```python
from build123d import *

# Parameters (mm, degrees)
F1_DEPTH = 12
F2_R     = 2.75
F3_DEPTH = 25
F4_R     = 4
F5_R     = 2
F6_R     = 1.6
F7_DEPTH = 25.001


with BuildPart() as f1:
    # F0 (on Top) → F1 (new body)
    with BuildSketch(Plane.XY):
        with BuildLine():
            ThreePointArc((1, 3.872983), (0, -4), (-1, 3.872983))
            Line((-1, 3.872983), (-1, 6.928203))
            Line((-1, 6.928203), (-1, 9.872983))
            Line((-1, 9.872983), (-5, 9.872983))
            Line((-5, 9.872983), (-5, 4.898979))
            ThreePointArc((-5, 4.898979), (-6.480741, 2.645751), (-7, 0))
            Line((-7, 0), (-7, -19))
            Line((-7, -19), (-20, -19))
            Line((-20, -19), (-20, -23))
            Line((-20, -23), (0, -23))
            Line((0, -23), (20, -23))
            Line((20, -23), (20, -19))
            Line((20, -19), (7, -19))
            Line((7, -19), (7, 0))
            ThreePointArc((7, 0), (6.480741, 2.645751), (5, 4.898979))
            Line((5, 4.898979), (5, 9.872983))
            Line((5, 9.872983), (1, 9.872983))
            Line((1, 9.872983), (1, 6.872983))
            Line((1, 6.872983), (1, 3.872983))
        make_face()
    extrude(amount=F1_DEPTH)

    # F2 (on face) → F3 (cut)
    with BuildSketch(Plane(origin=(0, -19, 0), x_dir=(-1, 0, 0), z_dir=(0, 1, 0))):
        with Locations((-13.5, 6)):
            Circle(F2_R)
        with Locations((13.5, 6)):
            Circle(F2_R)
    extrude(amount=-F3_DEPTH, mode=Mode.SUBTRACT)

    # F4
    f4_edges = [f1.edges().sort_by_distance(p)[0] for p in [
        (20, -21, 12),
        (20, -21, 0),
        (-20, -21, 0),
        (-20, -21, 12),
    ]]
    fillet(f4_edges, radius=F4_R)

    # F5
    f5_edges = [f1.edges().sort_by_distance(p)[0] for p in [
        (7, -19, 6),
        (-7, -19, 6),
    ]]
    fillet(f5_edges, radius=F5_R)

    # F6 (on face) → F7 (cut, through all)
    with BuildSketch(Plane.YZ.offset(5)):
        with Locations((7.385981, 6)):
            Circle(F6_R)
    extrude(amount=-F7_DEPTH, mode=Mode.SUBTRACT)


solid = f1.part
```
Geometry: final body of the model. Coordinates: model frame, mm. A direction names the side the tool comes from. Round coordinates to 2 decimals unless told otherwise and drop trailing zeros. Write each loop counter-clockwise with the first axis right and the second up, starting at its lowest first coordinate (ties: lowest second). Pieces come first, ordered by that corner, then holes.
Item 1: Section query B-B (z = 6). Give the number of separate pieces and of enclosed holes in the cut face, plus the area to 3 significant figures.
Item 2: Section query C-C (y = -1). Return loops of the section in (x, z), plus the area to 3 significant figures.
Item 3: Material intervals for L1, parallel to X at y = 0, z = 5.5; L2, parallel to Z at x = 13.5, y = -21.55; L3, parallel to X at y = 6, z = 1, sorted ascending.
Item 4: Section query D-D (x = 1.5). Return loops of the section in (y, z), plus the area to 3 significant figures.
Item 5: Mould query, pull axis X, two halves, no side actions, for faces 4 (the face through (1, 5.6, 5.9)), 5 (the face through (6.5, 2.6, 5.9)), 6 (the face through (0, -23, 6)), 7 (the face through (-1, 5, 6)). Classes: +X half, -X half, draft (parallel to the pull), parting line (faces both ways), or undercut.
Item 6: Section query A-A (x = 13.5). Return loops of the section in (y, z), plus the area to 3 significant figures.
Item 7: Set-up query: faces 1 (the face through (0, -10, 0)), 2 (the face through (17, -19, 6)), 3 (the face through (-5, 6.3, 4.6)). Return all of +Z, -Z, +X, -X, +Y, -Y with unobstructed straight access to the full face (end or side cutting, diameter ignored); none if empty.
Item 8: Pin query (flat end, axial travel): P1, Ø1.8, axis at y = 7.5, z = 8, coming from the -X side; P2, Ø1.5, axis at y = -4, z = 9.5, coming from the +X side; P3, Ø5.5, axis at x = -15, z = 5, coming from the +Y side. Return the tip coordinate at first contact, or that it passes through.
Completed:
1. separate pieces: 5
1. enclosed holes: 0
1. area: 408 mm2
2. outline: (-7, 0) - (-3.87, 0) - (-3.87, 12) - (-7, 12) - close; (3.87, 0) - (7, 0) - (7, 12) - (3.87, 12) - close
2. area: 75.0 mm2
3. L1: x = -7 to -4, 4 to 7
3. L2: z = 0 to 3.25, 8.75 to 12
3. L3: x = -5 to -1, 1 to 5
4. outline: (-23, 0) - (-3.71, 0) - (-3.71, 12) - (-23, 12) - close; (3.71, 0) - (9.87, 0) - (9.87, 12) - (3.71, 12) - close; hole circle Ø3.2 at (7.39, 6)
4. area: 297 mm2
5. face 4: undercut
5. face 5: +X half
5. face 6: draft
5. face 7: undercut
6. outline: (-23, 0) - (-19, 0) - (-19, 3.25) - (-23, 3.25) - close; (-23, 8.75) - (-19, 8.75) - (-19, 12) - (-23, 12) - close
6. area: 26.0 mm2
7. face 1: -Z, +X, -X, +Y, -Y
7. face 2: +Z, -Z, +X, +Y
7. face 3: +Z, -Z, -X, +Y
8. P1: stops at x = -5
8. P2: stops at x = 7
8. P3: stops at y = -19
